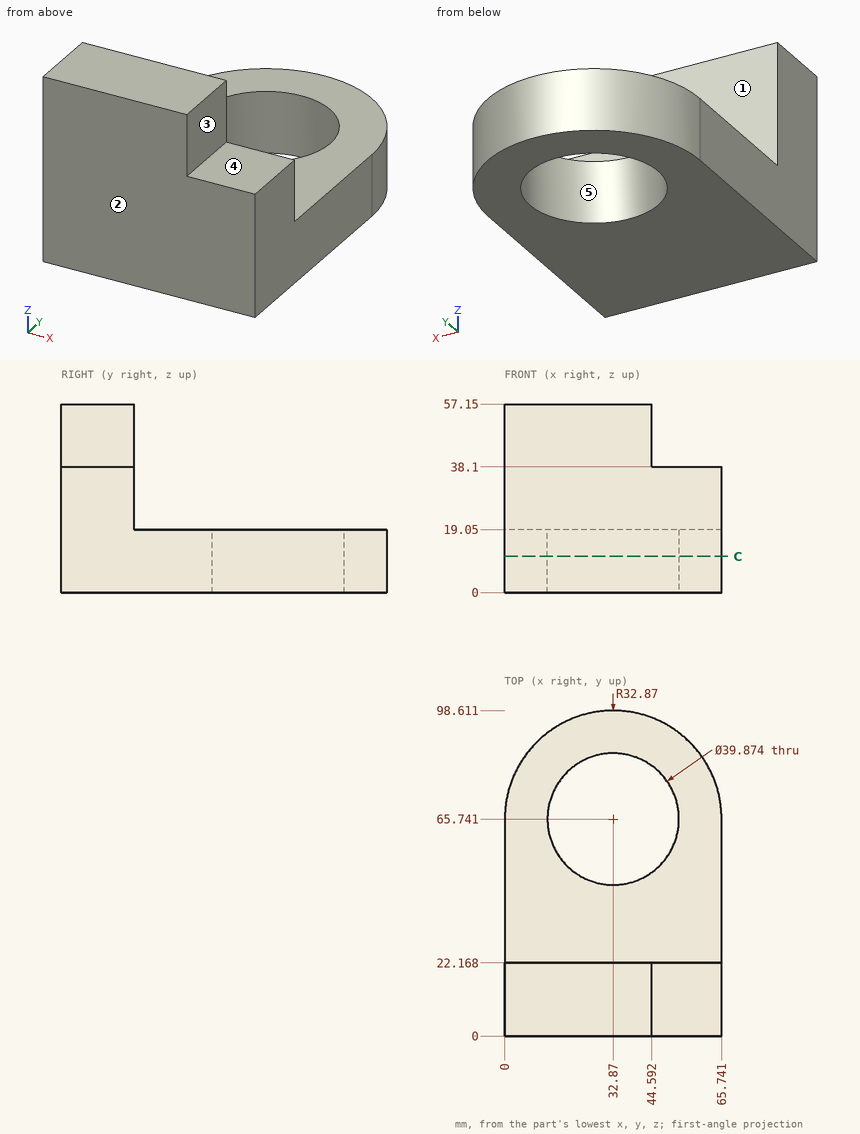
Here's the drawing with two shaded views (mm, measured from the low corner). I have some questions. A direction names the side the tool comes from. Give positions to 0.01 mm unless a question says otherwise; leave off trailing zeros. Order: outer loops, then holes, each group sorted by start corner. A loop starts at its lowest first (then second) coordinate and runs counter-clockwise, first axis right, second up. Notation, with made-up numbers: M -18.5,14.25 L -2.5,14.25 A21 ccw -2.5,39.25 Z; hole C 58,-29.5 d8. An arc over 180 degrees is marked long. One line per question, with ' | ' between items.
Item 1: Suppose I cut it at C-C, the plane z = 11. Write out the boundary of the cut face in (x, y), then the cut area to 3 significant figures.
Answer block:
outline: M 0,0 L 65.74,0 L 65.74,65.74 A32.87 ccw 0,65.74 Z; hole C 32.87,65.74 d39.87 | area: 4,770 mm2
Item 2: I'm going to push flat-ended pins straight in: pin 1 Ø12 at (x, y) = (28.5, 34) entering from +Z; pin 2 Ø15 at (y, z) = (13, 51) entering from +X; pin 3 Ø3 at (x, z) = (39.5, 10) entering from +Y. Where does each tip first touch, or does it pass through?
Answer block:
pin 1: stops at z = 19.05 | pin 2: stops at x = 44.59 | pin 3: stops at y = 98.21
Item 3: We'd pull the mould along X, two halves only. Please class the marked faces 3, 4 and 5: released by +X, released by -X, zero draft, split by the parting line, or undercut.
Answer block:
face 3: released by +X | face 4: zero draft | face 5: undercut
Item 4: Please list where these lines run through material, in increasing order: L1, parallel to Z at x = 46, y = 46.5; L2, parallel to Y at x = 15.5, z = 28.5; L3, parallel to Y at x = 50, z = 7.5 (1 decimal).
Answer block:
L1: z = 0 to 19.05 | L2: y = 0 to 22.17 | L3: y = 0 to 55.5, 75.9 to 93.8
Item 5: For the marked faces 1 and 2, which set-ups out of +Z, -Z, +X, -X, +Y, -Y let a thin tool reach every point of the face, with its end or its side?
Answer block:
face 1: +Z, +X, -X, +Y | face 2: +Z, -Z, +X, -X, -Y
